Build history of the part. All positions in model axes, mm. Face numbers are marked on the shaded views. A direction names the side the tool comes from. Coordinates: 2 decimals unless noted, no trailing zeros. Write each loop counter-clockwise with the first axis right and the second up, starting at its lowest first coordinate (ties: lowest second). Pieces come first, ordered by that corner, then holes. Notation, with made-up numbers: (-17.5, 62) -> (17.5, 62) arc R30 ccw to (17.5, 98) -> close; hole circle Ø8 at (81, 46.25). An arc over 180 degrees is marked (long way). Write each question's results on one line, items separated by ' | '. Start each with the question number.
Q1. Saw through at C-C on y = -11. Give the cut face in (x, z).
Q2. Drop flat-ended pins along their axis: pin 1 Ø2 at (x, y) = (-7.5, -11) entering from -Z; pin 2 Ø3 at (x, y) = (-11, -9) entering from +Z; pin 3 Ø2 at (x, y) = (5, -11) entering from -Z. Give the stop position or say it passes through.
Q3. Drill centre lines: line 1 (Z direction, x = 0, y = -4.5); line 2 (Y direction, x = 5.5, z = 8); line 3 (Z direction, x = 6, y = -3). Where is each one in solid material? Low to high.
Q4. Two-plate mould, pull along Z, no slides. Class the marked faces 3, 4 and 5: released by +Z, released by -Z, zero draft, split by the parting line, or undercut.
Q5. Saw through at A-A on z = 0. Give the cut face in (x, y), and give its area (3 significant figures).
Q6. Tool access for the marked faces 1 and 2: list every direction of +Z, -Z, +X, -X, +Y, -Y with a clear straight run to the whole face (end or side of a thin tool).
Q7. Saw through at B-B on x = 0. Give the cut face in (y, z).
from build123d import *

# Parameters (mm, degrees)
SKETCH1_R           = 17.5
BOSS_EXTRUDE1_DEPTH = 12.5
SKETCH2_R           = 15.9
CUT_EXTRUDE1_DEPTH  = 11
CHAMFER1_SIZE       = 2
CHAMFER2_SIZE       = 2


with BuildPart() as part:
    # Sketch1 → Boss-Extrude1 (new body)
    with BuildSketch(Plane(origin=(0, 0, 0), x_dir=(1, 0, 0), z_dir=(0, 1, 0))):
        Circle(SKETCH1_R)
    extrude(amount=-BOSS_EXTRUDE1_DEPTH)

    # Sketch2 → Cut-Extrude1 (cut)
    with BuildSketch(Plane.XZ.offset(12.5)):
        Circle(SKETCH2_R)
    extrude(amount=-CUT_EXTRUDE1_DEPTH, mode=Mode.SUBTRACT)

    # Chamfer1
    chamfer1_edges = [part.edges().sort_by_distance(p)[0] for p in [
        (-17.5, 0, 0),
    ]]
    chamfer(chamfer1_edges, length=CHAMFER1_SIZE)

    # Chamfer2
    chamfer2_edges = [part.edges().sort_by_distance(p)[0] for p in [
        (-15.9, -1.5, 0),
    ]]
    chamfer(chamfer2_edges, length=CHAMFER2_SIZE)


solid = part.part
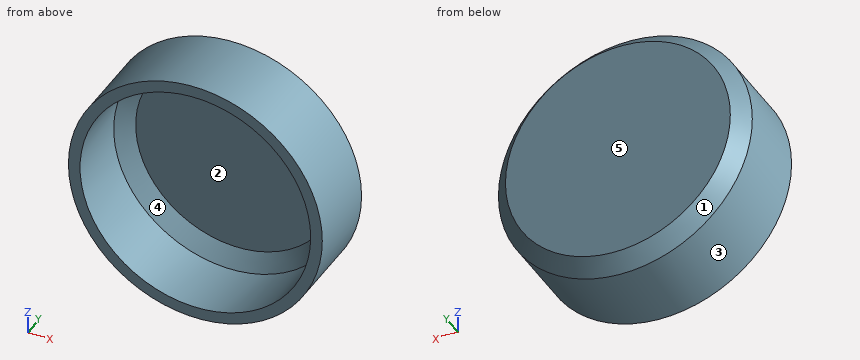
Returned:
1) outline: circle Ø35 at (0, 0); hole circle Ø31.8 at (0, 0)
2) pin 1: stops at z = -16.25 | pin 2: stops at z = 14.7 | pin 3: stops at z = -17.04
3) line 1: z = -17.5 to -15.9, 15.9 to 17.5 | line 2: y = -1.5 to 0 | line 3: z = -16.44 to -14.18, 14.18 to 16.44
4) face 3: split by the parting line | face 4: undercut | face 5: zero draft
5) outline: (-17.5, -12.5) -> (-15.9, -12.5) -> (-15.9, -3.5) -> (-13.9, -1.5) -> (13.9, -1.5) -> (15.9, -3.5) -> (15.9, -12.5) -> (17.5, -12.5) -> (17.5, -2) -> (15.5, 0) -> (-15.5, 0) -> (-17.5, -2) -> close | area: 87.7 mm2
6) face 1: +Y | face 2: -Y
7) outline: (-12.5, -17.5) -> (-2, -17.5) -> (0, -15.5) -> (0, 15.5) -> (-2, 17.5) -> (-12.5, 17.5) -> (-12.5, 15.9) -> (-3.5, 15.9) -> (-1.5, 13.9) -> (-1.5, -13.9) -> (-3.5, -15.9) -> (-12.5, -15.9) -> close
